```python
from build123d import *

# Parameters (mm, degrees)
SZKIC1_R                    = 5
DODANIE_WYCI_GNI_CIE1_DEPTH = 10


with BuildPart() as part:
    # Szkic1 → Dodanie-wyciągnięcie1 (new body)
    with BuildSketch(Plane(origin=(0, 0, 0), x_dir=(0, 0, -1), z_dir=(1, 0, 0))):
        Polygon((7.45669071, 15), (20, 2.45669071), (20, -15), (-20, -15), (-20, 15), align=None)
        with Locations((10, 0)):
            Circle(SZKIC1_R, mode=Mode.SUBTRACT)
    extrude(amount=DODANIE_WYCI_GNI_CIE1_DEPTH)


solid = part.part
```
Could you check a few things on this model? Use its own coordinates, in mm. Round coordinates to 2 decimals unless told otherwise and drop trailing zeros. Loops run counter-clockwise (first coordinate to the right, second up) from the corner with the lowest first, then second, coordinate; pieces in that order, holes last. Notation, with made-up numbers: M 59.5,13 L 107.5,13 A25 cw 107.5,39 Z; hole C 68,21.5 d6. An arc over 180 degrees is marked long. Answer as CSV lines item,"result".
1) Imagine slicing it at A-A on y = 0. List the corners of the cut face in (x, z) for me, and give its area (3 significant figures).
From the geometry:
outline,"M 0,-20 L 10,-20 L 10,-15 L 0,-15 Z; M 0,-5 L 10,-5 L 10,20 L 0,20 Z"
area,"300 mm^2"
2) Imagine slicing it at C-C on x = 2.25. List the corners of the cut face in (y, z) for me, and give its area (3 significant figures).
From the geometry:
outline,"M -15,-20 L 2.46,-20 L 15,-7.46 L 15,20 L -15,20 Z; hole C 0,-10 d10"
area,"1,040 mm^2"
3) We'd pull the mould along Z, two halves only. Please class faces 1 (the flat face through (5, 0, 20)), 2 (the cylindrical face through (4.93, 1.5, -14.77)), 3 (the flat face through (4.93, 8.816, -13.641)): released by +Z, released by -Z, zero draft, split by the parting line, or undercut.
From the geometry:
face 1,"released by +Z"
face 2,"undercut"
face 3,"released by -Z"
4) Imagine slicing it at D-D on y = 11.5. List the corners of the cut face in (x, z) for me.
From the geometry:
outline,"M 0,-10.96 L 10,-10.96 L 10,20 L 0,20 Z"
5) If I drill on probe 1 along Y at (x, z) = (2.25, -10); probe 2 along Z at (x, y) = (8, 1.5); probe 3 along Z at (x, y) = (5.5, -2.5), over which ranges is the centre line in solid material (lowest first)?
From the geometry:
probe 1,"-15 to -5, 5 to 12.46"
probe 2,"-20 to -14.77, -5.23 to 20"
probe 3,"-20 to -14.33, -5.67 to 20"
6) Imagine slicing it at B-B on z = -6. List the corners of the cut face in (x, y) for me.
From the geometry:
outline,"M 0,-15 L 10,-15 L 10,-3 L 0,-3 Z; M 0,3 L 10,3 L 10,15 L 0,15 Z"
